The model under review builds one solid part; all positions refer to its coordinate system, in mm. Give positions to 0.01 mm unless a question says otherwise; leave off trailing zeros. Loops run counter-clockwise (first coordinate to the right, second up) from the corner with the lowest first, then second, coordinate; pieces in that order, holes last. Notation, with made-up numbers: M -29.5,51 L 17.5,51 A23 cw 17.5,90 Z; hole C -31,37.25 d3. An arc over 180 degrees is marked long. Return JSON: item names as keys, results as strings.
```python
from build123d import *

# Parameters (mm, degrees)
BASPROSKE_W         = 3
BASPROSKE_H         = 14.625
TOOTHCUT_DEPTH      = 21.89931219
TEETHCUTS_COUNT     = 24
TEETHCUTS_ANGLE     = 345
BORSKE_R            = 1.5
BORE_DEPTH          = 50.0000508
SKETCH1_R           = 1.5
BOSS_EXTRUDE1_DEPTH = 3


with BuildPart() as part:
    # BasProSke → Base-Revolve (revolve)
    with BuildSketch(Plane(origin=(0, 0, 0), x_dir=(1, 0, 0), z_dir=(0, 1, 0)), mode=Mode.PRIVATE) as base_revolve_sk:
        with Locations((1.5, 7.3125)):
            Rectangle(BASPROSKE_W, BASPROSKE_H)
    revolve(base_revolve_sk.sketch.rotate(Axis((-10, 0, 0), (1, 0, 0)), 180), axis=Axis((-10, 0, 0), (1, 0, 0)))

    # TooCutSke → ToothCut (cut, through all)
    with BuildSketch(Plane(origin=(0, 0, 0), x_dir=(0, 0, -1), z_dir=(1, 0, 0))):
        with BuildLine():
            ThreePointArc((0.542722358, 12.080565177), (0, 12.09275), (-0.542722358, 12.080565177))
            ThreePointArc((-0.542722358, 12.080565177), (-0.922320579, 13.38903626), (-1.617327261, 14.56085412))
            ThreePointArc((-1.617327261, 14.56085412), (0, 14.6504), (1.617327261, 14.56085412))
            ThreePointArc((1.617327261, 14.56085412), (0.922320579, 13.38903626), (0.542722358, 12.080565177))
        make_face()
    toothcut = extrude(amount=TOOTHCUT_DEPTH, mode=Mode.SUBTRACT)

    # TeethCuts: ToothCut ×24 about axis
    teethcuts_axis = Axis((-10, 0, 0), (1, 0, 0))
    for i in range(1, TEETHCUTS_COUNT):
        add(toothcut.rotate(teethcuts_axis, i * TEETHCUTS_ANGLE / (TEETHCUTS_COUNT - 1)), mode=Mode.SUBTRACT)

    # BorSke → Bore (cut, symmetric)
    with BuildSketch(Plane(origin=(0, 0, 0), x_dir=(0, 0, -1), z_dir=(1, 0, 0))):
        with Locations(Location((0, 0, 0), (0, 0, 180))):
            Circle(BORSKE_R)
    extrude(amount=BORE_DEPTH, both=True, mode=Mode.SUBTRACT)

    # Sketch1 → Boss-Extrude1 (add)
    with BuildSketch(Plane(origin=(0, 0, 0), x_dir=(0, 0, -1), z_dir=(1, 0, 0))):
        with BuildLine():
            Line((31.167426359, -1.708998873), (11.983233878, 1.623794441))
            Line((11.983233878, 1.623794441), (10.733437515, -5.57027124))
            Line((10.733437515, -5.57027124), (29.917629996, -8.903064553))
            ThreePointArc((29.917629996, -8.903064553), (34.139561018, -5.930929895), (31.167426359, -1.708998873))
        make_face()
        with Locations((30.542528177, -5.306031713)):
            Circle(SKETCH1_R, mode=Mode.SUBTRACT)
    extrude(amount=BOSS_EXTRUDE1_DEPTH)


solid = part.part
```
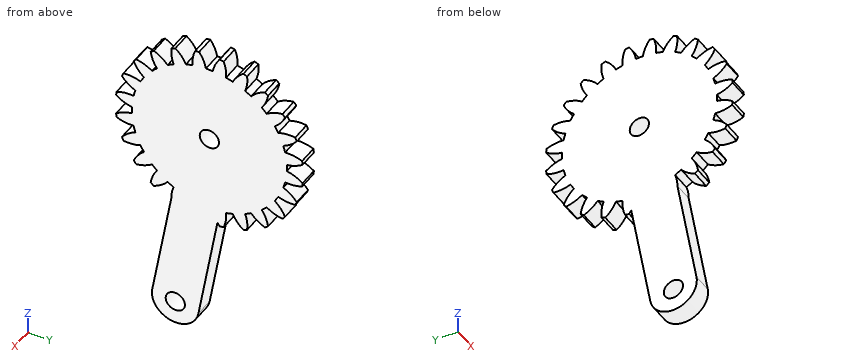
1) Consider section C-C on x = 0.5. Count the separate pieces of the cut face and the enclosed holes in it, then the cut area to 3 significant figures.
From the geometry:
{"separate pieces": "1", "enclosed holes": "2", "area": "693 mm²"}
2) Insertion check: pin 1 (2.5 mm diameter, centred on y = -5.31, z = -30.54, fed in from -X); pin 2 (1 mm diameter, centred on x = 1, z = 4.5, fed in from -Y). Each pin has a flat end and moves straight along its axis. Give the tip position at first contact, or say it passes through.
From the geometry:
{"pin 1": "through", "pin 2": "y = -13.37"}
3) Consider section A-A on z = 0. Write out the cut boundary in (x, y), then the cut area to 3 significant figures.
From the geometry:
{"outline": "M 0,-12.09 L 3,-12.09 L 3,-1.5 L 0,-1.5 Z; M 0,1.5 L 3,1.5 L 3,12.09 L 0,12.09 Z", "area": "63.6 mm²"}
4) Wall thickness on L1, parallel to Y at x = 1.8, z = 0; L2, parallel to Z at x = 0.2, y = 6.5; L3, parallel to Y at x = 1.8, z = -29.5: over which ranges is each line inside the solid? List them lowest first. Write a range as from..to.
From the geometry:
{"L1": "-12.09..-1.5, 1.5..12.09", "L2": "-10.2..10.2", "L3": "-8.83..-6.38, -4.23..-1.42"}
5) Consider section B-B on y = 0. Write out the cut boundary in (x, z).
From the geometry:
{"outline": "M 0,-21.33 L 3,-21.33 L 3,-1.5 L 0,-1.5 Z; M 0,1.5 L 3,1.5 L 3,12.09 L 0,12.09 Z"}
